The model under review builds one solid part; all positions refer to its coordinate system, in mm. Face numbers are marked on the shaded views. Coordinates: 2 decimals unless noted, no trailing zeros. Write each loop counter-clockwise with the first axis right and the second up, starting at its lowest first coordinate (ties: lowest second). Pieces come first, ordered by that corner, then holes.
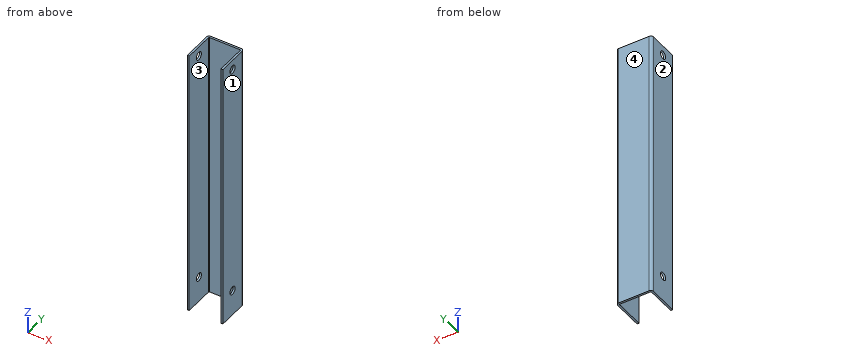
```python
from build123d import *

# Parameters (mm, degrees)
EKSTR_ZYON_NCE6_DEPTH                 = 420
M12_HELISARMAL_I_IN_Z_VANA_MATKAB_2_D = 12.25
M12_HELISARMAL_I_IN_Z_VANA_MATKAB_1_D = 12.25


with BuildPart() as part:
    # Çizim1 → Ekstrüzyon-İnce6 (new body)
    with BuildSketch(Plane.XY):
        with BuildLine():
            Line((-25.44311251, -27.126351083), (-25.44311251, 18.873648917))
            ThreePointArc((-25.44311251, 18.873648917), (-24.271539634, 21.702076041), (-21.44311251, 22.873648917))
            Line((-21.44311251, 22.873648917), (25.55688749, 22.873648917))
            ThreePointArc((25.55688749, 22.873648917), (28.385314615, 21.702076041), (29.55688749, 18.873648917))
            Line((29.55688749, 18.873648917), (29.55688749, -27.126351083))
            Line((29.55688749, -27.126351083), (26.55688749, -27.126351083))
            Line((26.55688749, -27.126351083), (26.55688749, 18.873648917))
            ThreePointArc((26.55688749, 18.873648917), (26.263994271, 19.580755698), (25.55688749, 19.873648917))
            Line((25.55688749, 19.873648917), (-21.44311251, 19.873648917))
            ThreePointArc((-21.44311251, 19.873648917), (-22.150219291, 19.580755698), (-22.44311251, 18.873648917))
            Line((-22.44311251, 18.873648917), (-22.44311251, -27.126351083))
            Line((-22.44311251, -27.126351083), (-25.44311251, -27.126351083))
        make_face()
    extrude(amount=EKSTR_ZYON_NCE6_DEPTH)

    # M12 Helisarmal için Zıvana matkabı2 (through all)
    with Locations(Plane.ZY.offset(25.44311251)):
        with Locations((40, -4.126351083)):
            Hole(M12_HELISARMAL_I_IN_Z_VANA_MATKAB_2_D / 2)

    # M12 Helisarmal için Zıvana matkabı1 (through all)
    with Locations(Plane.ZY.offset(25.44311251)):
        with Locations((405, -4.126351083)):
            Hole(M12_HELISARMAL_I_IN_Z_VANA_MATKAB_1_D / 2)


solid = part.part
```
Item 1: Mouldability with a two-part tool opening along X and no side actions: class the marked faces 1, 2, 3 and 4 as pulls with the +X half, pulls with the -X half, needs draft (parallel to the pull), parting line crosses it, or undercut.
Solved:
face 1: pulls with the +X half
face 2: pulls with the -X half
face 3: undercut
face 4: needs draft
Item 2: To check wall thickness, follow line 1 along X through (y, z) = (11.5, 130); line 2 along Y through (x, z) = (15.5, 241); line 3 along Y through (x, z) = (-24, 405). State the ranges of each line that lie inside material, in increasing order.
Solved:
line 1: x = -25.44 to -22.44, 26.56 to 29.56
line 2: y = 19.87 to 22.87
line 3: y = -27.13 to -10.25, 2 to 21.95
Item 3: Take a section at D-D, the plane x = 19.5. Write out the cut boundary in (y, z), plus the area to 3 significant figures.
Solved:
outline: (19.87, 0) - (22.87, 0) - (22.87, 420) - (19.87, 420) - close
area: 1,260 mm2
Item 4: Take a section at C-C, the plane z = 209. Write out the cut boundary in (x, y), plus the area to 3 significant figures.
Solved:
outline: (-25.44, -27.13) - (-22.44, -27.13) - (-22.44, 18.87) arc R1 cw to (-21.44, 19.87) - (25.56, 19.87) arc R1 cw to (26.56, 18.87) - (26.56, -27.13) - (29.56, -27.13) - (29.56, 18.87) arc R4 ccw to (25.56, 22.87) - (-21.44, 22.87) arc R4 ccw to (-25.44, 18.87) - close
area: 441 mm2
Item 5: Take a section at B-B, the plane z = 405. Write out the cut boundary in (x, y), plus the area to 3 significant figures.
Solved:
outline: (-25.44, -27.13) - (-22.44, -27.13) - (-22.44, -10.25) - (-25.44, -10.25) - close; (-25.44, 2) - (-22.44, 2) - (-22.44, 18.87) arc R1 cw to (-21.44, 19.87) - (25.56, 19.87) arc R1 cw to (26.56, 18.87) - (26.56, 2) - (29.56, 2) - (29.56, 18.87) arc R4 ccw to (25.56, 22.87) - (-21.44, 22.87) arc R4 ccw to (-25.44, 18.87) - close; (26.56, -27.13) - (29.56, -27.13) - (29.56, -10.25) - (26.56, -10.25) - close
area: 367 mm2
Item 6: For pin 1 (1.5 mm diameter, centred on x = 17.5, z = 42, fed in from -Y); pin 2 (16 mm diameter, centred on y = -4.13, z = 405, fed in from +X), all flat-tipped, find the tip position at first contact; note any pin that passes through.
Solved:
pin 1: stops at y = 19.87
pin 2: stops at x = 29.56
Item 7: Take a section at A-A, the plane y = 7. Write out the cut boundary in (x, z), plus the area to 3 significant figures.
Solved:
outline: (-25.44, 0) - (-22.44, 0) - (-22.44, 420) - (-25.44, 420) - close; (26.56, 0) - (29.56, 0) - (29.56, 420) - (26.56, 420) - close
area: 2,520 mm2
